Verification items for the finished model (mm, model axes). Face numbers are marked on the shaded views. Coordinates: 2 decimals unless noted, no trailing zeros. Write each loop counter-clockwise with the first axis right and the second up, starting at its lowest first coordinate (ties: lowest second). Pieces come first, ordered by that corner, then holes. Notation, with made-up numbers: (17, 44) -> (32, 44) arc R21 ccw to (32, 65) -> close; hole circle Ø9 at (-19.75, 69.25). An arc over 180 degrees is marked (long way). Answer in a Markdown table with one row per item.
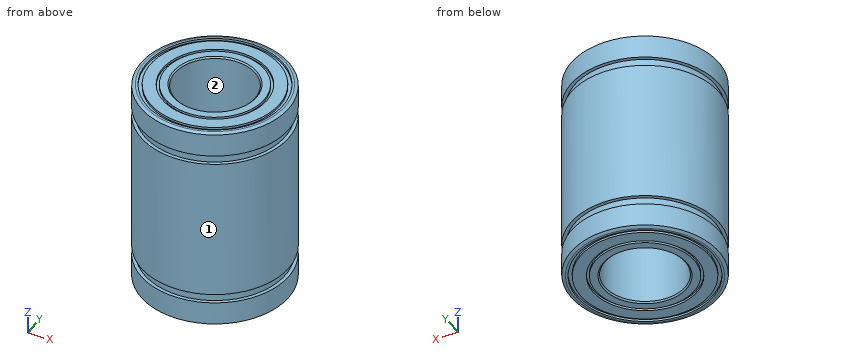
```python
from build123d import *


with BuildPart() as part:
    # Sketch1 → Revolve1 (revolve)
    with BuildSketch(Plane.XZ, mode=Mode.PRIVATE) as revolve1_sk:
        Polygon((6.495238095, 15.714285714), (6.285714286, 15.504761905), (6.285714286, -15.504761905), (6.495238095, -15.714285714), (7.637142857, -15.714285714), (7.637142857, -15.384285714), (8.049642857, -15.384285714), (8.049642857, -15.714285714), (9.9, -15.714285714), (9.9, -15.384285714), (10.45, -15.384285714), (10.45, -15.714285714), (10.79047619, -15.714285714), (11.285714286, -15.504761905), (11.285714286, -12.047619048), (10.761904762, -12.047619048), (10.761904762, -10.685714286), (11.285714286, -10.685714286), (11.285714286, 10.685714286), (10.761904762, 10.685714286), (10.761904762, 12.047619048), (11.285714286, 12.047619048), (11.285714286, 15.504761905), (10.79047619, 15.714285714), (10.45, 15.714285714), (10.45, 15.384285714), (9.9, 15.384285714), (9.9, 15.714285714), (8.049642857, 15.714285714), (8.049642857, 15.384285714), (7.637142857, 15.384285714), (7.637142857, 15.714285714), align=None)
    revolve(revolve1_sk.sketch.rotate(Axis((0.285714286, 0, 15.714285714), (0, 0, -1)), 270), axis=Axis((0.285714286, 0, 15.714285714), (0, 0, -1)))


solid = part.part
```
1. Go/stop test with flat-tipped pins: pin 1 (4 mm diameter, centred on x = -2.5, z = 2.5, fed in from +Y); pin 2 (1 mm diameter, centred on x = -5.5, z = -10, fed in from -Y); pin 3 (1 mm diameter, centred on y = 1.5, z = 1.5, fed in from +X). Record where each tip stops, or that it passes through.
Findings below:
| item | result |
|---|---|
| pin 1 | stops at y = 10.97 |
| pin 2 | stops at y = -9.65 |
| pin 3 | stops at x = 11.24 |
2. Sectioned sample at A-A, the plane z = 9. Record the cut outline in (x, y), and give its area (3 significant figures).
Findings below:
| item | result |
|---|---|
| outline | circle Ø22 at (0.29, 0); hole circle Ø12 at (0.29, 0) |
| area | 267 mm² |
3. Material ranges on probe 1 along X at (y, z) = (0, -15.45); probe 2 along Z at (x, y) = (-8.5, 6.5); probe 3 along X at (y, z) = (0, -15.55), recorded low to high. Write a range as from..to.
Findings below:
| item | result |
|---|---|
| probe 1 | x = -10.71..-9.88, -9.33..-7.48, -7.07..-5.71, 6.29..7.64, 8.05..9.9, 10.45..11.29 |
| probe 2 | z = -15.53..-12.05, -10.69..10.69, 12.05..15.53 |
| probe 3 | x = -10.61..-9.88, -9.33..-7.48, -7.07..-5.76, 6.33..7.64, 8.05..9.9, 10.45..11.18 |
4. Release check for a two-part mould opening along X. For the marked faces 1 and 2 record: released by +X, released by -X, zero draft, split by the parting line, or undercut.
Findings below:
| item | result |
|---|---|
| face 1 | split by the parting line |
| face 2 | undercut |
